Input: dimensioned drawing with shaded views. Units: mm. Origin: part minimum x, y, z. A direction names the side the tool comes from. Round coordinates to 2 decimals unless told otherwise and drop trailing zeros. Loops run counter-clockwise (first coordinate to the right, second up) from the corner with the lowest first, then second, coordinate; pieces in that order, holes last. Notation, with made-up numbers: M 41,36.25 L 97,36.25 A18 ccw 97,64.25 Z; hole C 73,73.5 d9. An arc over 180 degrees is marked long. Put each result on its own line as item: value. Start each with the question number.
1) Section D-D on y = 74.5. Output: boundary loops of the cut face in (x, z), plus the area to 3 significant figures.
2) Section C-C on x = 19. Output: boundary loops of the cut face in (y, z).
3) Line query: probe 1 along X at (y, z) = (28, 18.5); probe 2 along Y at (x, z) = (36, 3); probe 3 along Y at (x, z) = (28.5, 35). Output: solid intervals per line, ascending.
4) Reachability of the marked faces 1, 2, 3, 4 and 5 from +Z, -Z, +X, -X, +Y, -Y: full face, straight path, thin tool, end or side. Return the list, or none.
5) Section B-B on z = 37. Output: boundary loops of the cut face in (x, y), plus the area to 3 significant figures.
6) Section A-A on y = 22. Output: boundary loops of the cut face in (x, z).
7) Pin query (flat end, axial travel): pin 1 (9 mm diameter, centred on y = 74, z = 13.5, fed in from +X); pin 2 (2 mm diameter, centred on y = 69.5, z = 14, fed in from -X); pin 3 (8 mm diameter, centred on x = 5, y = 59.5, fed in from +Z); pin 4 (4.5 mm diameter, centred on x = 5, z = 11, fed in from +Y). Return the tip coordinate at first contact, or that it passes through.
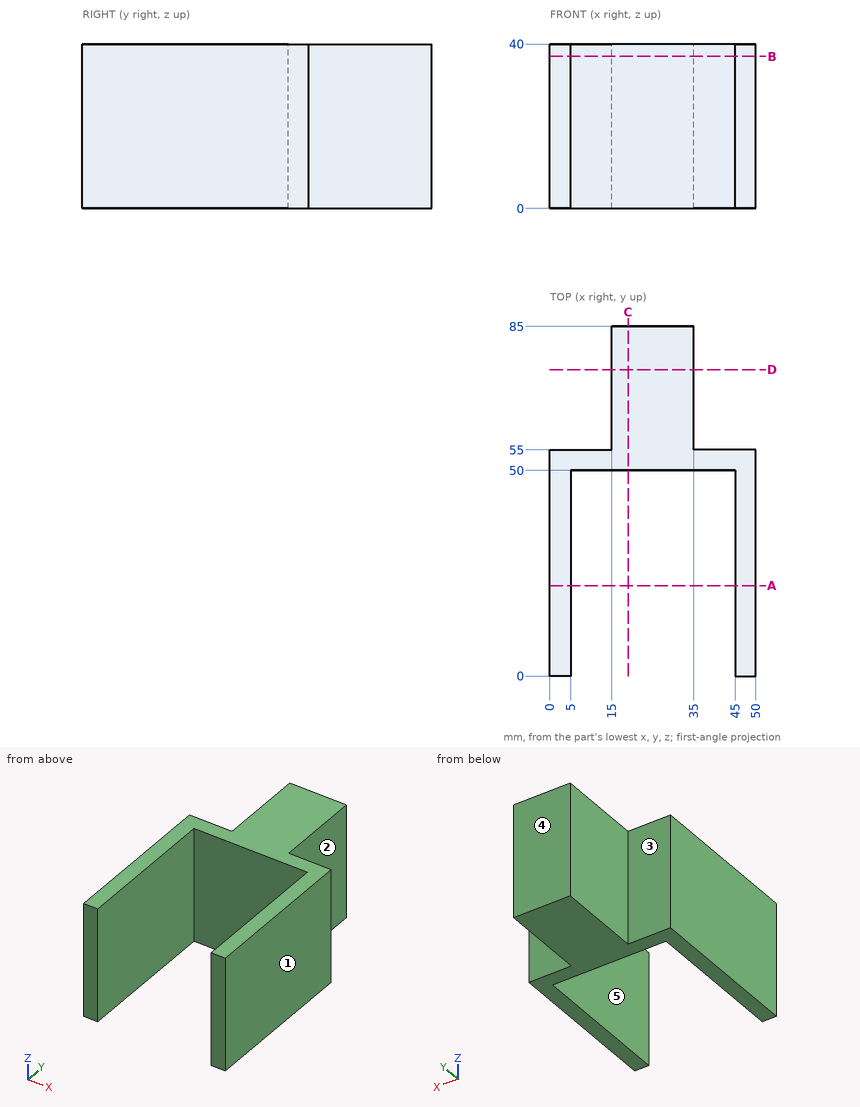
Geometry results:
1. outline: M 15,0 L 35,0 L 35,40 L 15,40 Z
1. area: 800 mm²
2. outline: M 50,0 L 85,0 L 85,40 L 50,40 Z
3. probe 1: x = 0 to 5, 45 to 50
3. probe 2: y = 50 to 55
3. probe 3: y = 50 to 85
4. face 1: +Z, -Z, +X, +Y, -Y
4. face 2: +Z, -Z, +X, +Y
4. face 3: +Z, -Z, -X, +Y
4. face 4: +Z, -Z, +X, -X, +Y
4. face 5: +Z, -Z, -Y
5. outline: M 0,0 L 5,0 L 5,50 L 45,50 L 45,0 L 50,0 L 50,55 L 35,55 L 35,85 L 15,85 L 15,55 L 0,55 Z
5. area: 1,350 mm²
6. outline: M 0,0 L 5,0 L 5,40 L 0,40 Z; M 45,0 L 50,0 L 50,40 L 45,40 Z
7. pin 1: stops at x = 35
7. pin 2: stops at x = 15
7. pin 3: passes through
7. pin 4: stops at y = 55
